```python
from build123d import *

# Parameters (mm, degrees)
BOSS_EXTRUDE1_DEPTH       = 25
SKETCH2_R                 = 3
BOSS_EXTRUDE2_DEPTH       = 9
F_6_0MM_DOWEL_HOLE1_D     = 6
F_6_0MM_DOWEL_HOLE1_DEPTH = 9
F_6_0MM_DOWEL_HOLE1_TIP   = 1.802581857


with BuildPart() as part:
    # Sketch1 → Boss-Extrude1 (new body)
    with BuildSketch(Plane(origin=(0, 0, 0), x_dir=(1, 0, 0), z_dir=(0, 1, 0))):
        Polygon((7.505553499, 0), (3.75277675, 6.5), (-3.75277675, 6.5), (-7.505553499, 0), (-3.75277675, -6.5), (3.75277675, -6.5), align=None)
    extrude(amount=BOSS_EXTRUDE1_DEPTH)

    # Sketch2 → Boss-Extrude2 (add)
    with BuildSketch(Plane.XZ):
        with Locations(Location((0, 0, 0), (0, 0, 90))):
            Circle(SKETCH2_R)
    extrude(amount=BOSS_EXTRUDE2_DEPTH)

    # Ø6.0mm Dowel Hole1
    with Locations(Plane(origin=(0, 25, 0), x_dir=(1, 0, 0), z_dir=(0, 1, 0))):
        with Locations((0, 0)):
            Hole(F_6_0MM_DOWEL_HOLE1_D / 2, depth=F_6_0MM_DOWEL_HOLE1_DEPTH)
            with Locations((0, 0, -(F_6_0MM_DOWEL_HOLE1_DEPTH + F_6_0MM_DOWEL_HOLE1_TIP / 2))):  # 118° drill point
                Cone(0, F_6_0MM_DOWEL_HOLE1_D / 2, F_6_0MM_DOWEL_HOLE1_TIP, mode=Mode.SUBTRACT)


solid = part.part
```
Design review of the part built by this model. Coordinates are the model's own, in mm. A direction names the side the tool comes from. Give positions to 0.01 mm unless a question says otherwise; leave off trailing zeros. Order: outer loops, then holes, each group sorted by start corner. A loop starts at its lowest first (then second) coordinate and runs counter-clockwise, first axis right, second up. Notation, with made-up numbers: (-3.75, -28.75) -> (11.25, -28.75) arc R20 ccw to (11.25, -21.75) -> close; hole circle Ø8 at (30, -30.5). An arc over 180 degrees is marked (long way). Write each question's results on one line, items separated by ' | '. Start each with the question number.
Q1. Machinability: for faces 5 (the flat face through (3.2, 0, -0.1)), 6 (the flat face through (5.66, 12.32, -3.2)), 7 (the cylindrical face through (3, 20, 0)), which of the approach directions +Z, -Z, +X, -X, +Y, -Y give a long, thin tool a straight path to every point of the face, cutting with its end or side? Answer none if there is none.
Q2. Add section B-B on y = 7.5. Give the boundary of the cut face in (x, z).
Q3. Wall thickness on L1, parallel to Z at x = 0, y = 20; L2, parallel to Y at x = -5.25, z = -2.5; L3, parallel to Z at x = -2.75, y = 22.5: over which ranges is each line inside the solid? List them lowest first. Write a range as from..to.
Q4. Add section C-C on x = -5. Give the boundary of the cut face in (y, z), and give its area (3 significant figures).
Q5. Mouldability with a two-part tool opening along Z and no side actions: class faces 1 (the conical face through (-0.11, 14.51, 0.51)), 2 (the cylindrical face through (-0.9, -4.44, 2.86)), 3 (the flat face through (3.2, 25, -0.1)), 4 (the flat face through (0, 12, -6.5)) as +Z half, -Z half, draft (parallel to the pull), parting line (faces both ways), or undercut.
Q6. Add section D-D on y = 15. Give the boundary of the cut face in (x, z), and give its area (3 significant figures).
Q7. For pin 1 (5 mm diameter, centred on y = 1, z = 3.5, fed in from -X); pin 2 (6 mm diameter, centred on y = -5.5, z = 2, fed in from -X); pin 3 (1 mm diameter, centred on x = 2.5, z = 3, fed in from -Y); pin 4 (3 mm diameter, centred on y = -4, z = 5, fed in from -X), all flat-tipped, find the tip position at first contact; note any pin that passes through.
Q8. Add section A-A on y = 21.5. Give the boundary of the cut face in (x, z), and give its area (3 significant figures).
Found:
1) face 5: -Y | face 6: -Z, +X, +Y, -Y | face 7: +Y
2) outline: (-7.51, 0) -> (-3.75, -6.5) -> (3.75, -6.5) -> (7.51, 0) -> (3.75, 6.5) -> (-3.75, 6.5) -> close
3) L1: z = -6.5..-3, 3..6.5 | L2: y = 0..25 | L3: z = -6.5..-1.2, 1.2..6.5
4) outline: (0, -4.34) -> (25, -4.34) -> (25, 4.34) -> (0, 4.34) -> close | area: 217 mm2
5) face 1: undercut | face 2: parting line | face 3: draft | face 4: -Z half
6) outline: (-7.51, 0) -> (-3.75, -6.5) -> (3.75, -6.5) -> (7.51, 0) -> (3.75, 6.5) -> (-3.75, 6.5) -> close; hole circle Ø2.67 at (0, 0) | area: 141 mm2
7) pin 1: stops at x = -6.93 | pin 2: stops at x = -3 | pin 3: stops at y = 0 | pin 4: passes through
8) outline: (-7.51, 0) -> (-3.75, -6.5) -> (3.75, -6.5) -> (7.51, 0) -> (3.75, 6.5) -> (-3.75, 6.5) -> close; hole circle Ø6 at (0, 0) | area: 118 mm2
